```python
from build123d import *

# Parameters (mm, degrees)
BOSS_EXTRUDE2_DEPTH = 12


with BuildPart() as part:
    # Sketch1 → Boss-Extrude2 (new body)
    with BuildSketch(Plane.XY):
        Polygon((0, 250), (0, 0), (150, 0), (150, 27.638698422), (30, 250), align=None)
        with BuildLine():
            Line((21, 15), (129.719822185, 15))
            ThreePointArc((129.719822185, 15), (134.872349516, 17.925676968), (135, 23.849512632))
            Line((135, 23.849512632), (26.280177815, 225.308522369))
            ThreePointArc((26.280177815, 225.308522369), (19.530487647, 228.276271415), (15, 222.459009736))
            Line((15, 222.459009736), (15, 21))
            ThreePointArc((15, 21), (16.757359313, 16.757359313), (21, 15))
        make_face(mode=Mode.SUBTRACT)
    extrude(amount=BOSS_EXTRUDE2_DEPTH)


solid = part.part
```
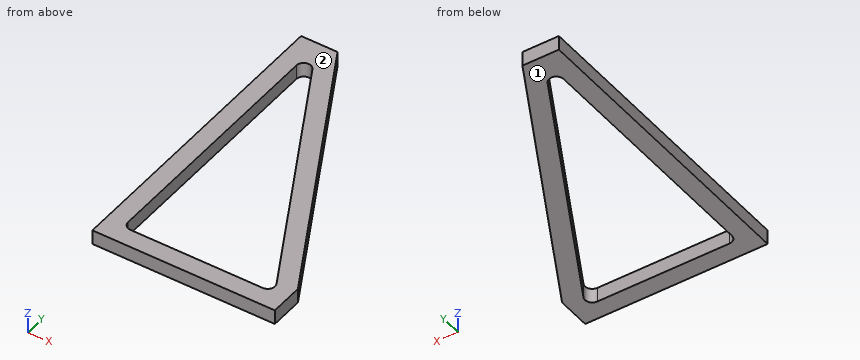
Read the model definition and answer for the solid it produces. Units are mm, in the model's axes. Face numbers are marked on the shaded views. Give positions to 0.01 mm unless a question says otherwise; leave off trailing zeros. Loops run counter-clockwise (first coordinate to the right, second up) from the corner with the lowest first, then second, coordinate; pieces in that order, holes last.
Item 1: Each of these flat-tipped pins is pushed along its axis until it touches: pin 1 Ø6 at (y, z) = (217, 6.5) entering from +X; pin 2 Ø3 at (y, z) = (144, 6) entering from +X. Where does it stop, or does it pass through?
Item 2: Find the intervals of material crossed by line 1 along X through (y, z) = (62, 7.25); line 2 along X through (y, z) = (145.5, 0.5); line 3 along Y through (x, z) = (50, 1.25), in increasing order.
Item 3: The part is cut by section B-B (y = 85). Write down the section's boundary in (x, z).
Item 4: The mould has two halves that part along Z. Classify the marked faces 1 and 2: released by +Z, released by -Z, zero draft, split by the parting line, or undercut.
Item 5: The part is cut by section A-A (x = 43). Write down the section's boundary in (y, z).
Taken from the geometry:
1. pin 1: stops at x = 49.43
1. pin 2: stops at x = 88.01
2. line 1: x = 0 to 15, 114.41 to 131.46
2. line 2: x = 0 to 15, 69.35 to 86.39
2. line 3: y = 0 to 15, 181.36 to 212.94
3. outline: (0, 0) - (15, 0) - (15, 12) - (0, 12) - close; (102, 0) - (119.04, 0) - (119.04, 12) - (102, 12) - close
4. face 1: released by -Z
4. face 2: released by +Z
5. outline: (0, 0) - (15, 0) - (15, 12) - (0, 12) - close; (194.33, 0) - (225.91, 0) - (225.91, 12) - (194.33, 12) - close
